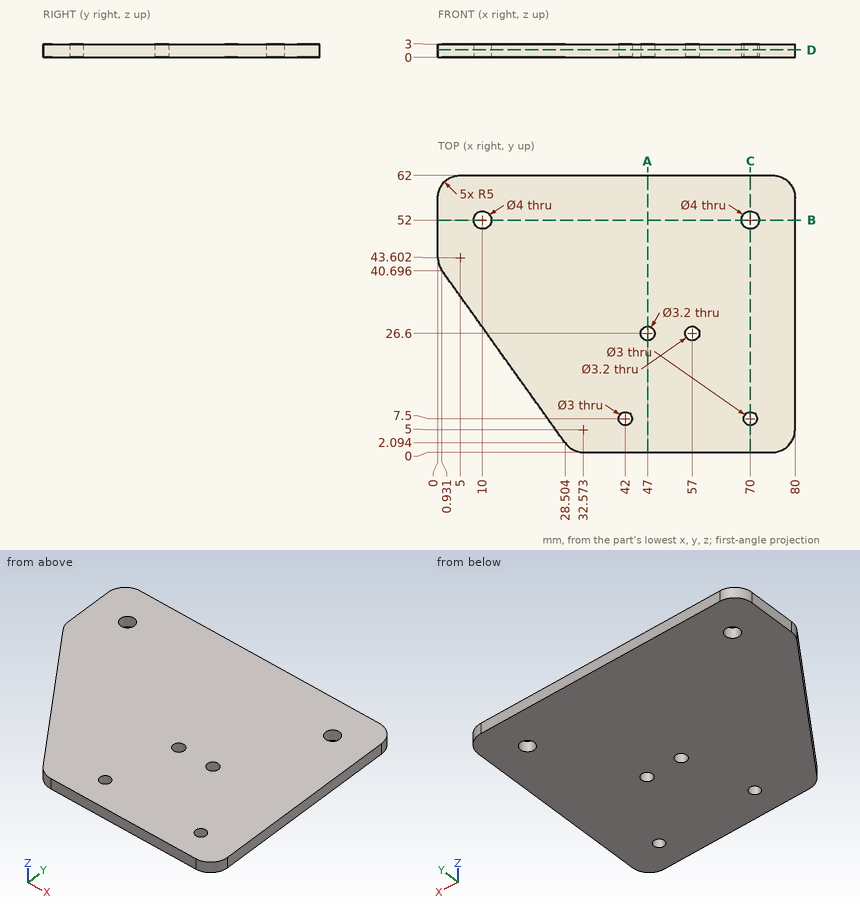
Design review of the part shown in the three views and the two pictorial views. Dimensions are in mm from the part's minimum x, y and z. Coordinates: 2 decimals unless noted, no trailing zeros. Write each loop counter-clockwise with the first axis right and the second up, starting at its lowest first coordinate (ties: lowest second). Pieces come first, ordered by that corner, then holes.
1) Clearance check with flat-ended pins moving along their axes: pin 1 Ø3.5 at (x, y) = (57, 26.6) entering from -Z; pin 2 Ø3 at (x, y) = (47, 26.6) entering from -Z. State where each tip first meets the part, or that it passes through.
2) We need section D-D on z = 1.7. State the section outline as (x, y) points (1 decimal), then the cut area to 3 significant figures.
3) We need section B-B on y = 52. State the section outline as (x, z) points, then the cut area to 3 significant figures.
4) To check wall thickness, follow probe 1 along Y at (x, z) = (70, 1.1); probe 2 along Y at (x, z) = (42, 2.45); probe 3 along Y at (x, z) = (47, 0.8). State the ranges of each line that lie inside material, in increasing order.
5) We need section A-A on x = 47. State the section outline as (y, z) points.
6) We need section C-C on x = 70. State the section outline as (y, z) points.
Answer list:
1. pin 1: stops at z = 0
1. pin 2: passes through
2. outline: (0, 43.6) arc R5 ccw to (0.9, 40.7) - (28.5, 2.1) arc R5 ccw to (32.6, 0) - (75, 0) arc R5 ccw to (80, 5) - (80, 57) arc R5 ccw to (75, 62) - (5, 62) arc R5 ccw to (0, 57) - close; hole circle Ø4 at (10, 52); hole circle Ø3 at (42, 7.5); hole circle Ø3.2 at (47, 26.6); hole circle Ø3.2 at (57, 26.6); hole circle Ø4 at (70, 52); hole circle Ø3 at (70, 7.5)
2. area: 4,260 mm2
3. outline: (0, 0) - (8, 0) - (8, 3) - (0, 3) - close; (12, 0) - (68, 0) - (68, 3) - (12, 3) - close; (72, 0) - (80, 0) - (80, 3) - (72, 3) - close
3. area: 216 mm2
4. probe 1: y = 0 to 6, 9 to 50, 54 to 62
4. probe 2: y = 0 to 6, 9 to 62
4. probe 3: y = 0 to 25, 28.2 to 62
5. outline: (0, 0) - (25, 0) - (25, 3) - (0, 3) - close; (28.2, 0) - (62, 0) - (62, 3) - (28.2, 3) - close
6. outline: (0, 0) - (6, 0) - (6, 3) - (0, 3) - close; (9, 0) - (50, 0) - (50, 3) - (9, 3) - close; (54, 0) - (62, 0) - (62, 3) - (54, 3) - close
